The model under review builds one solid part; all positions refer to its coordinate system, in mm. Round coordinates to 2 decimals unless told otherwise and drop trailing zeros. Order: outer loops, then holes, each group sorted by start corner. A loop starts at its lowest first (then second) coordinate and runs counter-clockwise, first axis right, second up. Notation, with made-up numbers: M 44.25,-7 L 90.25,-7 A11 ccw 90.25,9 Z; hole C 24.5,75.25 d6. An arc over 180 degrees is marked long. Use a Markdown table: item, result. Add a question column.
1. To check wall thickness, follow probe 1 along Y at (x, z) = (139, 0.3); probe 2 along X at (y, z) = (73, 1.9); probe 3 along Y at (x, z) = (110.5, 3). State the ranges of each line that lie inside material, in increasing order.
2. Consider section C-C on x = 187. State the section outline as (y, z) points (3 decimals), then the cut area to 3 significant figures.
3. Consider section A-A on x = 29. State the section outline as (y, z) points (3 decimals).
4. Insertion check: P1, Ø1.7, axis at y = 44, z = 2.5, coming from the +X side; P2, Ø3, axis at x = 12, z = 2, coming from the -Y side. Each pin has a flat end and moves straight along its axis. Give the tip position at first contact, or say it passes through.
5. Consider section D-D on x = 86. State the section outline as (y, z) points (3 decimals), then the cut area to 3 significant figures.
6. Consider section B-B on z = 1.7. Count the separate pieces of the cut face and the enclosed holes in it, then the cut area to 3 significant figures.
from build123d import *

# Parameters (mm, degrees)
BOSS_EXTRUDE1_DEPTH = 5.715


with BuildPart() as part:
    # Model → Boss-Extrude1 (new body)
    with BuildSketch(Plane.XY):
        Polygon((16.114776, 23.2006394), (38.974776, 23.2006394), (39.713662, 23.2006394), (41.932098, 23.590631), (44.254166, 24.4808502), (44.689776, 24.7316498), (45.123862, 24.983821), (47.05604, 26.54935), (48.622712, 28.481274), (48.87341, 28.91536), (49.124362, 29.350716), (50.690018, 31.282894), (52.621688, 32.848296), (53.057044, 33.098994), (53.491384, 33.349946), (55.813198, 34.241486), (58.031888, 34.630106), (58.772044, 34.630106), (223.458532, 34.630106), (224.197418, 34.630106), (226.415854, 34.241486), (228.737922, 33.349946), (229.173278, 33.098994), (229.60711, 32.848296), (231.539288, 31.282894), (233.104944, 29.350716), (233.355388, 28.91536), (233.60634, 28.481274), (235.171996, 26.54935), (237.103666, 24.983821), (237.539276, 24.7316498), (237.973362, 24.4808502), (240.2967, 23.590631), (242.51539, 23.2006394), (243.255546, 23.2006394), (266.11326, 23.2006394), (266.11326, 30.64891), (271.8308, 30.64891), (271.8308, 42.078402), (266.11326, 42.078402), (266.11326, 53.509418), (271.8308, 53.509418), (271.8308, 64.938656), (266.11326, 64.938656), (266.11326, 76.060554), (262.46074, 80.41386), (266.8397, 84.087716), (259.49148, 92.844112), (255.11252, 89.170256), (247.767094, 97.926144), (252.145038, 101.6), (244.797326, 110.355888), (240.419382, 106.682032), (233.073194, 115.438428), (237.451138, 119.112284), (230.103426, 127.868172), (225.725482, 124.194316), (218.37904, 132.950204), (222.757238, 136.62406), (215.409272, 145.378932), (211.031328, 141.7066), (207.3783, 146.060922), (195.283328, 146.060922), (195.283328, 151.775668), (183.852312, 151.775668), (183.852312, 146.060922), (172.423074, 146.060922), (172.423074, 151.775668), (160.993328, 151.775668), (160.993328, 146.060922), (149.562566, 146.060922), (149.562566, 151.775668), (138.133328, 151.775668), (138.133328, 146.060922), (126.702312, 146.060922), (126.702312, 151.775668), (115.273074, 151.775668), (115.273074, 146.060922), (103.843328, 146.060922), (103.843328, 151.775668), (92.412566, 151.775668), (92.412566, 146.060922), (80.983328, 146.060922), (80.983328, 151.775668), (69.552312, 151.775668), (69.552312, 146.060922), (58.123074, 146.060922), (58.123074, 151.775668), (46.693328, 151.775668), (46.693328, 146.060922), (35.262566, 146.060922), (35.262566, 151.775668), (23.8331756, 151.775668), (23.8331756, 146.060922), (16.114776, 146.060922), (16.114776, 136.066022), (10.4000554, 136.066022), (10.4000554, 124.63526), (16.114776, 124.63526), (16.114776, 113.205768), (10.4000554, 113.205768), (10.4000554, 101.775006), (16.114776, 101.775006), (16.114776, 90.345768), (10.4000554, 90.345768), (10.4000554, 78.916022), (16.114776, 78.916022), (16.114776, 67.48526), (10.4000554, 67.48526), (10.4000554, 56.055768), (16.114776, 56.055768), (16.114776, 44.625006), (10.4000554, 44.625006), (10.4000554, 33.195514), (16.114776, 33.195514), align=None)
        Polygon((26.815288, 40.346122), (21.1005166, 40.346122), (21.1005166, 46.060868), (32.530034, 46.060868), (32.530034, 40.346122), align=None, mode=Mode.SUBTRACT)
        Polygon((49.675796, 40.346122), (43.959272, 40.346122), (43.959272, 46.060868), (55.390288, 46.060868), (55.390288, 40.346122), align=None, mode=Mode.SUBTRACT)
        Polygon((72.534272, 40.346122), (66.819526, 40.346122), (66.819526, 46.060868), (78.250796, 46.060868), (78.250796, 40.346122), align=None, mode=Mode.SUBTRACT)
        Polygon((95.394526, 40.346122), (89.680034, 40.346122), (89.680034, 46.060868), (101.109272, 46.060868), (101.109272, 40.346122), align=None, mode=Mode.SUBTRACT)
        Polygon((118.255034, 40.346122), (112.540288, 40.346122), (112.540288, 46.060868), (123.969526, 46.060868), (123.969526, 40.346122), align=None, mode=Mode.SUBTRACT)
        Polygon((141.115288, 40.346122), (135.400796, 40.346122), (135.400796, 46.060868), (146.830034, 46.060868), (146.830034, 40.346122), align=None, mode=Mode.SUBTRACT)
        Polygon((163.975796, 40.346122), (158.259272, 40.346122), (158.259272, 46.060868), (169.690288, 46.060868), (169.690288, 40.346122), align=None, mode=Mode.SUBTRACT)
        Polygon((186.834272, 40.346122), (181.119526, 40.346122), (181.119526, 46.060868), (192.550796, 46.060868), (192.550796, 40.346122), align=None, mode=Mode.SUBTRACT)
        Polygon((209.694526, 40.346122), (203.980034, 40.346122), (203.980034, 46.060868), (215.409272, 46.060868), (215.409272, 40.346122), align=None, mode=Mode.SUBTRACT)
        Polygon((232.555034, 40.346122), (226.840288, 40.346122), (226.840288, 46.060868), (238.269526, 46.060868), (238.269526, 40.346122), align=None, mode=Mode.SUBTRACT)
        Polygon((255.41478, 40.346122), (249.700796, 40.346122), (249.700796, 46.060868), (261.12978, 46.060868), (261.12978, 40.346122), align=None, mode=Mode.SUBTRACT)
    extrude(amount=BOSS_EXTRUDE1_DEPTH)


solid = part.part
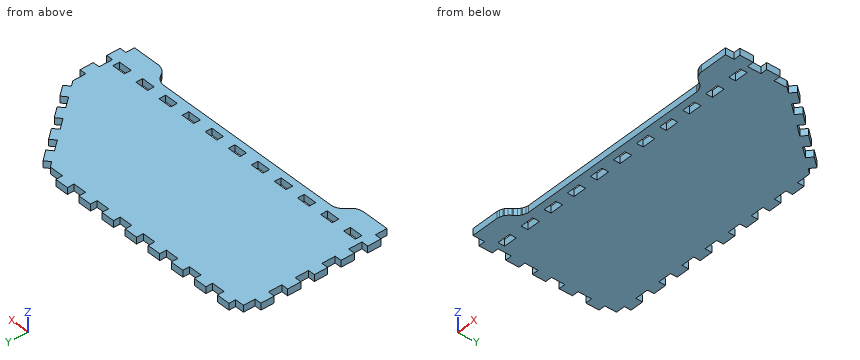
Answer block:
| question | item | result |
|---|---|---|
| 1 | probe 1 | 34.63 to 40.35, 46.06 to 151.78 |
| 1 | probe 2 | 16.11 to 266.11 |
| 1 | probe 3 | 34.63 to 146.06 |
| 2 | outline | M 34.63,0 L 40.346,0 L 40.346,5.715 L 34.63,5.715 Z; M 46.061,0 L 151.776,0 L 151.776,5.715 L 46.061,5.715 Z |
| 2 | area | 637 mm^2 |
| 3 | outline | M 23.201,0 L 40.346,0 L 40.346,5.715 L 23.201,5.715 Z; M 46.061,0 L 151.776,0 L 151.776,5.715 L 46.061,5.715 Z |
| 4 | P1 | x = 266.11 |
| 4 | P2 | y = 33.2 |
| 5 | outline | M 34.63,0 L 146.061,0 L 146.061,5.715 L 34.63,5.715 Z |
| 5 | area | 637 mm^2 |
| 6 | separate pieces | 1 |
| 6 | enclosed holes | 11 |
| 6 | area | 27,100 mm^2 |
